Can you work these out from the model? Positions are in its coordinate system, mm. A direction names the side the tool comes from. Give positions to 0.01 mm unless a question says otherwise; leave off trailing zeros. Write each loop counter-clockwise with the first axis right and the second up, starting at its lowest first coordinate (ties: lowest second). Pieces come first, ordered by that corner, then holes.
from build123d import *
from build123d.topology import SkipClean

# Parameters (mm, degrees)
SZKIC1_W                        = 20
SZKIC1_H                        = 52.3
SZKIC1_R                        = 2.8
DODANIE_WYCI_GNI_CIE1_DEPTH     = 22
SZKIC2_R                        = 4.8
WYTNIJ_WYCI_GNI_CIE1_DEPTH      = 7
ZAOKR_GLENIE1_R                 = 8
WYTNIJ_WYCI_GNI_CIE2_DEPTH      = 161.813163879
WYTNIJ_WYCI_GNI_CIE2_DEPTH_BACK = 161.813163879
WYTNIJ_WYCI_GNI_CIE3_REACH      = 163.032
SZKIC7_R                        = 2.8
DODANIE_WYCI_GNI_CIE2_DEPTH     = 0.2
SFAZOWANIE1_SIZE                = 3
SFAZOWANIE2_SIZE                = 3
ZAOKR_GLENIE2_R                 = 10
SFAZOWANIE3_SIZE                = 0.8
ZAOKR_GLENIE3_START             = -102
ZAOKR_GLENIE3_DEPTH             = 6.947286026
ZAOKR_GLENIE3_START_2           = 51
ZAOKR_GLENIE3_2_DEPTH           = 6.499237843


with BuildPart() as part:
    # Szkic1 → Dodanie-wyciągnięcie1 (new body)
    with BuildSketch(Plane.XY):
        with Locations((-31.301196691, 132.11386567)):
            Rectangle(SZKIC1_W, SZKIC1_H)
        with Locations((-31.301196691, 148.26386567)):
            Circle(SZKIC1_R, mode=Mode.SUBTRACT)
        with Locations(Location((-31.301196691, 115.96386567, 0), (0, 0, 180))):
            Circle(SZKIC1_R, mode=Mode.SUBTRACT)
        Polygon((-33.860213685, 125.96386567), (-39.063328725, 125.96386567), (-39.451196691, 126.351733636), (-39.451196691, 137.875997705), (-39.063328725, 138.26386567), (-33.860213685, 138.26386567), (-33.560213685, 138.26386567), (-33.042179696, 138.26386567), (-32.742179696, 138.26386567), (-31.539064656, 138.26386567), (-31.151196691, 137.875997705), (-31.151196691, 126.351733636), (-31.539064656, 125.96386567), (-32.742179696, 125.96386567), (-33.042179696, 125.96386567), (-33.560213685, 125.96386567), align=None, mode=Mode.SUBTRACT)
    extrude(amount=DODANIE_WYCI_GNI_CIE1_DEPTH)

    # Szkic2 → Wytnij-wyciągnięcie1 (cut)
    with BuildSketch(Plane.XY.offset(22)):
        with Locations((-31.301196691, 148.26386567)):
            Circle(SZKIC2_R)
        with Locations((-31.301196691, 115.81386567)):
            Circle(SZKIC2_R)
    extrude(amount=-WYTNIJ_WYCI_GNI_CIE1_DEPTH, mode=Mode.SUBTRACT)

    # Zaokrąglenie1
    zaokr_glenie1_edges = [part.edges().sort_by_distance(p)[0] for p in [
        (-41.301196691, 105.96386567, 11),
        (-41.301196691, 158.26386567, 11),
        (-21.301196691, 158.26386567, 11),
        (-21.301196691, 105.96386567, 11),
    ]]
    fillet(zaokr_glenie1_edges, radius=ZAOKR_GLENIE1_R)

    # Szkic4 → Wytnij-wyciągnięcie2 (cut, two sides: drawn at the far end of the back side and taken through both)
    with BuildSketch(Plane(origin=(-39.451196691, 0, 0), x_dir=(0, 0, -1), z_dir=(1, 0, 0)).offset(-WYTNIJ_WYCI_GNI_CIE2_DEPTH_BACK)):
        with BuildLine():
            Line((-13.5, 133.61386567), (-11.5, 133.61386567))
            ThreePointArc((-11.5, 133.61386567), (-10, 132.11386567), (-11.5, 130.61386567))
            Line((-11.5, 130.61386567), (-13.5, 130.61386567))
            ThreePointArc((-13.5, 130.61386567), (-15, 132.11386567), (-13.5, 133.61386567))
        make_face()
    extrude(amount=WYTNIJ_WYCI_GNI_CIE2_DEPTH + WYTNIJ_WYCI_GNI_CIE2_DEPTH_BACK, mode=Mode.SUBTRACT)

    # Szkic6 → Wytnij-wyciągnięcie3 (cut, up to next)
    with BuildSketch(Plane.ZY.offset(41.301196691), mode=Mode.PRIVATE) as wytnij_wyci_gni_cie3_sk1:
        with BuildLine():
            Line((11.5, 128.61386567), (13.5, 128.61386567))
            ThreePointArc((13.5, 128.61386567), (17, 132.11386567), (13.5, 135.61386567))
            Line((13.5, 135.61386567), (11.5, 135.61386567))
            ThreePointArc((11.5, 135.61386567), (8, 132.11386567), (11.5, 128.61386567))
        make_face()
    wytnij_wyci_gni_cie3_tool1 = extrude(wytnij_wyci_gni_cie3_sk1.sketch, amount=-WYTNIJ_WYCI_GNI_CIE3_REACH, mode=Mode.PRIVATE) & part.part
    add(wytnij_wyci_gni_cie3_tool1.solids().sort_by_distance((-41.301197, 132.113866, 12.5))[0], mode=Mode.SUBTRACT)

    # Szkic7 → Dodanie-wyciągnięcie2 (add)
    with BuildSketch(Plane(origin=(0, 0, 0), x_dir=(-1, 0, 0), z_dir=(0, 0, -1))):
        with Locations((31.301196691, 115.96386567)):
            Circle(SZKIC7_R)
        with Locations((31.301196691, 148.26386567)):
            Circle(SZKIC7_R)
        Polygon((31.539064656, 125.96386567), (31.151196691, 126.351733636), (31.151196691, 137.875997705), (31.539064656, 138.26386567), (39.063328725, 138.26386567), (39.451196691, 137.875997705), (39.451196691, 126.351733636), (39.063328725, 125.96386567), align=None)
    extrude(amount=-DODANIE_WYCI_GNI_CIE2_DEPTH)

    # Sfazowanie1
    # the kernel refuses this chamfer: 3 mm, written as the material it takes off along each edge
    with BuildSketch(Plane(origin=(-21.301196691, 157.978914634, 22), x_dir=(0, 0, -1), z_dir=(0, -1, 0))) as sfazowanie1_piece_1:
        Polygon((SFAZOWANIE1_SIZE, 0), (0, -SFAZOWANIE1_SIZE), (0, 0), align=None)
    extrude(amount=51.730097928, mode=Mode.SUBTRACT)

    # Sfazowanie2
    # the kernel refuses this chamfer: 3 mm, written as the material it takes off along each edge
    with BuildSketch(Plane(origin=(-21.586147727, 105.96386567, 22), x_dir=(0, 1, 0), z_dir=(-1, 0, 0)), Plane(origin=(-41.016245655, 158.26386567, 22), x_dir=(0, -1, 0), z_dir=(1, 0, 0))) as sfazowanie2_piece_1:
        Polygon((SFAZOWANIE2_SIZE, 0), (0, SFAZOWANIE2_SIZE), (0, 0), align=None)
    extrude(amount=19.430097928, mode=Mode.SUBTRACT)

    # Zaokrąglenie2
    zaokr_glenie2_edges = [part.edges().sort_by_distance(p)[0] for p in [
        (-23.972769566, 108.635438546, 21.671572875),
        (-23.972769566, 155.592292795, 21.671572875),
    ]]
    fillet(zaokr_glenie2_edges, radius=ZAOKR_GLENIE2_R)

    # Sfazowanie3
    sfazowanie3_edges = [part.edges().sort_by_distance(p)[0] for p in [
        (-40.849705947, 152.913395441, 22),
        (-40.849705947, 111.3143359, 22),
        (-41.301196691, 132.11386567, 22),
    ]]
    chamfer(sfazowanie3_edges, length=SFAZOWANIE3_SIZE)

    # Zaokrąglenie3: read off the stored shape, not the designer's step
    # Zaokrąglenie3 outline → Zaokrąglenie3 (cut)
    with SkipClean():  # the faces are left unmerged after this step: merging them gives an invalid solid
        with BuildSketch(Plane(origin=(0, 0, 0), x_dir=(0.8164965809277239, 0.4082482904638656, -0.40824829046386485), z_dir=(0.5773502691896288, -0.5773502691896248, 0.5773502691896238)).offset(ZAOKR_GLENIE3_START)):
            with BuildLine():
                ThreePointArc((18.448905373, 120.344481475), (22.109159411, 124.004735513), (27.109159411, 125.344481475))
                Line((27.109159411, 125.344481475), (17, 125.344481475))
                Line((17, 125.344481475), (17, 119))
                Line((17, 119), (17.672668632, 119))
                Line((17.672668632, 119), (18.448905373, 120.344481475))
            make_face()
        extrude(amount=ZAOKR_GLENIE3_DEPTH, mode=Mode.SUBTRACT)

    # Zaokr_glenie3 2 outline → Zaokr_glenie3 2 (cut)
    with BuildSketch(Plane(origin=(0, 0, 0), x_dir=(0.816496580927723, -0.4082482904638645, -0.40824829046386735), z_dir=(0.5773502691896298, 0.5773502691896218, 0.5773502691896258)).offset(ZAOKR_GLENIE3_START_2)):
        with BuildLine():
            Line((-91, 61.492739134), (-80.761360202, 61.492739134))
            ThreePointArc((-80.761360202, 61.492739134), (-85.761360202, 62.832485096), (-89.42161424, 66.492739134))
            Line((-89.42161424, 66.492739134), (-90.291831707, 68))
            Line((-90.291831707, 68), (-91, 68))
            Line((-91, 68), (-91, 61.492739134))
        make_face()
    extrude(amount=ZAOKR_GLENIE3_2_DEPTH, mode=Mode.SUBTRACT)


solid = part.part
(1) If I drill on L1, parallel to Z at x = -24.75, y = 132; L2, parallel to Y at x = -30.25, z = 10.75; L3, parallel to Y at x = -36, z = 7.25, over which ranges is the centre line in solid material (lowest first)?
Returned:
L1: z = 0 to 10, 15 to 22
L2: y = 105.96 to 113.37, 118.56 to 130.81, 133.41 to 145.67, 150.86 to 158.26
L3: y = 106.43 to 125.96, 138.26 to 157.79
(2) Imagine slicing it at B-B, the plane z = 7.25. Write out the boundary of the cut face in (x, y).
Returned:
outline: (-41.3, 113.96) arc R8 ccw to (-33.3, 105.96) - (-29.3, 105.96) arc R8 ccw to (-21.3, 113.96) - (-21.3, 150.26) arc R8 ccw to (-29.3, 158.26) - (-33.3, 158.26) arc R8 ccw to (-41.3, 150.26) - close; hole (-39.45, 126.35) - (-39.06, 125.96) - (-31.54, 125.96) - (-31.15, 126.35) - (-31.15, 137.88) - (-31.54, 138.26) - (-39.06, 138.26) - (-39.45, 137.88) - close; hole circle Ø5.6 at (-31.3, 115.96); hole circle Ø5.6 at (-31.3, 148.26)
(3) Imagine slicing it at C-C, the plane y = 144. Write out the boundary of the cut face in (x, z).
Returned:
outline: (-41.3, 0) - (-21.3, 0) - (-21.3, 19) - (-24.3, 22) - (-29.1, 22) - (-29.1, 15) - (-33.51, 15) - (-33.51, 22) - (-40.5, 22) - (-41.3, 21.2) - close
(4) If we mould it in two halves opening along Y, with no side actions, what happens to faces 3 (the face through (-25.09, 154.58, 20.84)), 4 (the face through (-31, 132, 0)), 5 (the face through (-26.3, 132.1, 10))? For each: +Y half, -Y half, draft (parallel to the pull), parting line (faces both ways), or undercut.
Returned:
face 3: +Y half
face 4: draft
face 5: undercut
(5) Imagine slicing it at A-A, the plane z = 16.5. Write out the boundary of the cut face in (x, y).
Returned:
outline: (-41.3, 113.96) arc R8 ccw to (-33.3, 105.96) - (-29.3, 105.96) arc R8 ccw to (-21.3, 113.96) - (-21.3, 150.26) arc R8 ccw to (-29.3, 158.26) - (-33.3, 158.26) arc R8 ccw to (-41.3, 150.26) - (-41.3, 133.92) - (-39.45, 133.92) - (-39.45, 137.88) - (-39.06, 138.26) - (-31.54, 138.26) - (-31.15, 137.88) - (-31.15, 126.35) - (-31.54, 125.96) - (-39.06, 125.96) - (-39.45, 126.35) - (-39.45, 130.31) - (-41.3, 130.31) - close; hole circle Ø9.6 at (-31.3, 115.81); hole circle Ø9.6 at (-31.3, 148.26)
(6) Will these pins go through, and if not, where does the flat tip stop? P1, Ø6, axis at x = -31, y = 149, coming from the +Z side; P2, Ø0.6, axis at x = -24.5, z = 12, coming from the -Y side; P3, Ø2, axis at x = -40.5, z = 12.5, coming from the +Y side.
Returned:
P1: stops at z = 15
P2: stops at y = 107.35
P3: stops at y = 155.32
(7) For faces 1 (the face through (-29, 146, 15)), 2 (the face through (-23.707, 155.983, 9.86)), which set-ups out of +Z, -Z, +X, -X, +Y, -Y let a thin tool reach every point of the face, with its end or its side?
Returned:
face 1: +Z
face 2: +Z, -Z, +X, +Y
